Verification items for the finished model (mm, model axes). A direction names the side the tool comes from. Round coordinates to 2 decimals unless told otherwise and drop trailing zeros. Write each loop counter-clockwise with the first axis right and the second up, starting at its lowest first coordinate (ties: lowest second). Pieces come first, ordered by that corner, then holes. Notation, with made-up numbers: (-25.5, 65.25) - (-3.5, 65.25) arc R8 ccw to (-3.5, 77.25) - close; hole circle Ø6 at (51, -23.5). An arc over 180 degrees is marked (long way). Answer as a JSON object with one key per item and string values. Group by question number.
1) Thickness scan on line 1 (Z direction, x = 0, y = -49); line 2 (X direction, y = -94.5, z = 10); line 3 (X direction, y = -93, z = 7.5). Record the ranges inside material, lowest first.
2) Section check A-A (x = 0). Enter the section's corners in (y, z).
3) Mould release check, pull along X, two halves, no side actions. Record for faces 1 (the flat face through (8, -101.6, -25)), 2 (the cylindrical face through (-5.506, -51.511, -24.796)), 3 (the flat face through (76.2, -25, -1)), 4 (the cylindrical face through (-30.235, -75.844, -23.183)): +X half, -X half, draft (parallel to the pull), parting line (faces both ways), or undercut.
4) Section check D-D (y = -65). Enter the section's corners in (x, z).
5) Go/stop test with a flat-tipped pin: pin 1 Ø12 at (y, z) = (-58.5, 9) entering from +X. Record where the tip stops, or that it passes through.
6) Section check C-C (z = 19.5). Enter the section's corners in (x, y), then the cut area to 3 significant figures.
7) Set-up check for faces 5 (the flat face through (-1, -25, -50.8)), 6 (the flat face through (-18, -50.8, 35)): record each of +Z, -Z, +X, -X, +Y, -Y from which the full face is reachable in a straight line by a thin tool's end or side.
8) Section check B-B (y = -36.5). Enter the section's corners in (x, z).
```python
from build123d import *

# Parameters (mm, degrees)
F0_W     = 152.4
F0_H     = 101.6
F1_DEPTH = 50.8
F3_R     = 38.1
F4_DEPTH = 50.8
F5_R     = 25.4
F6_DEPTH = 101.6


with BuildPart() as f1:
    # F0 (on Front) → F1 (new body)
    with BuildSketch(Plane.XZ):
        Rectangle(F0_W, F0_H)
    extrude(amount=F1_DEPTH)

    # F3 (on face) → F4 (join)
    with BuildSketch(Plane.XZ.offset(50.8)):
        Circle(F3_R)
    extrude(amount=F4_DEPTH)

    # F5 (on face) → F6 (cut)
    with BuildSketch(Plane.XZ.offset(101.6)):
        Circle(F5_R)
    extrude(amount=-F6_DEPTH, mode=Mode.SUBTRACT)


solid = f1.part
```
Returned:
{
 "1": {"line 1": "-50.8 to -25.4, 25.4 to 50.8", "line 2": "-36.76 to -23.35, 23.35 to 36.76", "line 3": "-37.35 to -24.27, 24.27 to 37.35"},
 "2": {"outline": "(-101.6, -38.1) - (-50.8, -38.1) - (-50.8, -50.8) - (0, -50.8) - (0, -25.4) - (-101.6, -25.4) - close; (-101.6, 25.4) - (0, 25.4) - (0, 50.8) - (-50.8, 50.8) - (-50.8, 38.1) - (-101.6, 38.1) - close"},
 "3": {"face 1": "draft", "face 2": "undercut", "face 3": "+X half", "face 4": "parting line"},
 "4": {"outline": "circle Ø76.2 at (0, 0); hole circle Ø50.8 at (0, 0)"},
 "5": {"pin 1": "x = 37.98"},
 "6": {"outline": "(-76.2, -50.8) - (-32.73, -50.8) - (-32.73, -101.6) - (-16.28, -101.6) - (-16.28, 0) - (-76.2, 0) - close; (16.28, -101.6) - (32.73, -101.6) - (32.73, -50.8) - (76.2, -50.8) - (76.2, 0) - (16.28, 0) - close", "area": "7,760 mm2"},
 "7": {"face 5": "-Z, +X, -X, +Y, -Y", "face 6": "-Y"},
 "8": {"outline": "(-76.2, -50.8) - (76.2, -50.8) - (76.2, 50.8) - (-76.2, 50.8) - close; hole circle Ø50.8 at (0, 0)"}
}
